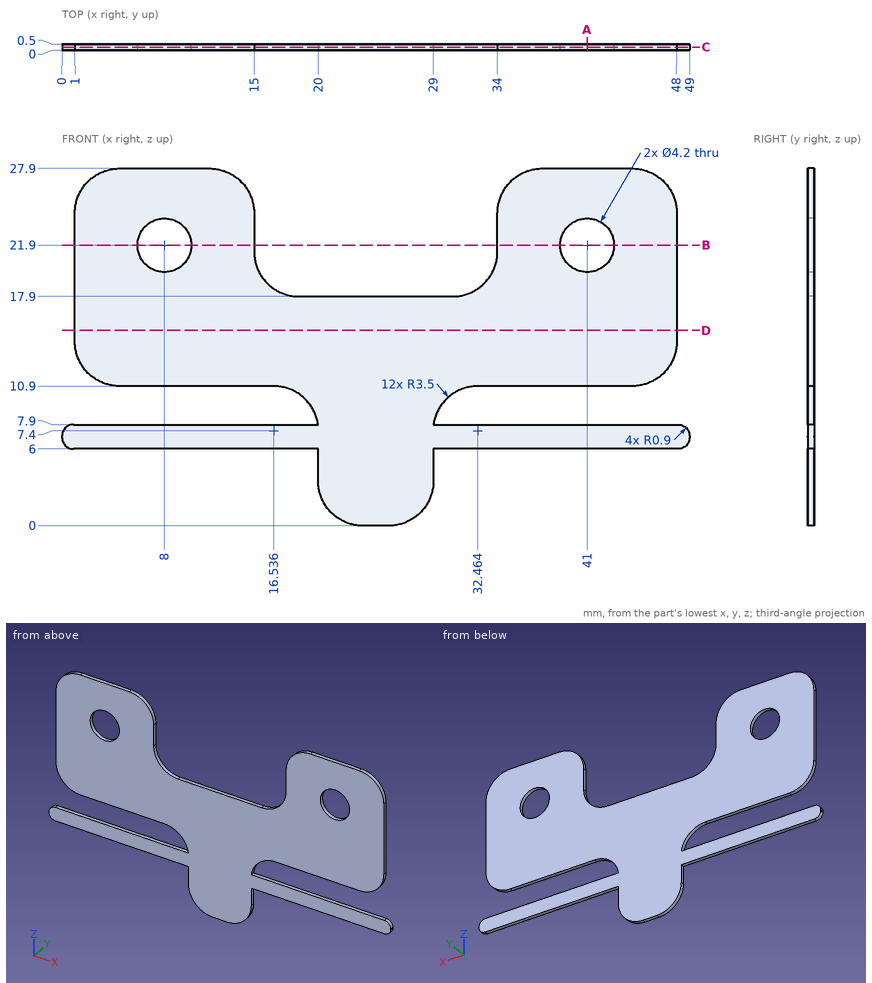
Here's the drawing with two shaded views (mm, measured from the low corner). I have some questions. Give positions to 0.01 mm unless a question says otherwise; leave off trailing zeros. Write each loop counter-clockwise with the first axis right and the second up, starting at its lowest first coordinate (ties: lowest second). Pieces come first, ordered by that corner, then holes. Notation, with made-up numbers: (-19, 3) - (33, 3) arc R36 cw to (33, 39) - close; hole circle Ø6 at (66.25, 18). An arc over 180 degrees is marked (long way). One line per item, written item: value. Start each with the question number.
Item 1: Imagine slicing it at C-C, the plane y = 0.25. Give the number of separate pieces and of enclosed holes in the cut face, and give its area (3 significant figures).
Item 2: Imagine slicing it at D-D, the plane z = 15.25. List the corners of the cut face in (x, y) for me.
Item 3: Imagine slicing it at B-B, the plane z = 21.9. List the corners of the cut face in (x, y) for me.
Item 4: Please list where these lines run through material, in increasing order: line 1 (X direction, y = 0.4, z = 21.9); line 2 (Z direction, x = 8, y = 0.45); line 3 (Z direction, x = 11.5, y = 0.2). Write a range as from..to.
Item 5: Imagine slicing it at A-A, the plane x = 41. List the corners of the cut face in (y, z) for me.
Item 6: I'm going to push a flat-ended pin straight in: pin 1 (5.5 mm diameter, centred on x = 8, z = 21.9, fed in from -Y). Where does the tip first touch, or does it pass through?
Geometry says:
1. separate pieces: 1
1. enclosed holes: 2
1. area: 744 mm^2
2. outline: (1, 0) - (48, 0) - (48, 0.5) - (1, 0.5) - close
3. outline: (1, 0) - (5.9, 0) - (5.9, 0.5) - (1, 0.5) - close; (10.1, 0) - (15, 0) - (15, 0.5) - (10.1, 0.5) - close; (34, 0) - (38.9, 0) - (38.9, 0.5) - (34, 0.5) - close; (43.1, 0) - (48, 0) - (48, 0.5) - (43.1, 0.5) - close
4. line 1: 1..5.9, 10.1..15, 34..38.9, 43.1..48
4. line 2: 6..7.9, 10.9..19.8, 24..27.9
4. line 3: 6..7.9, 10.9..27.9
5. outline: (0, 6) - (0.5, 6) - (0.5, 7.9) - (0, 7.9) - close; (0, 10.9) - (0.5, 10.9) - (0.5, 19.8) - (0, 19.8) - close; (0, 24) - (0.5, 24) - (0.5, 27.9) - (0, 27.9) - close
6. pin 1: y = 0
